```python
from build123d import *

# Parameters (mm, degrees)
F0_R     = 1.9
F1_DEPTH = 8
F2_R     = 2.9
F3_DEPTH = 10
F5_W     = 18.789151
F5_H     = 32.01971
F6_DEPTH = 25


with BuildPart() as f1:
    # F0 (on Top) → F1 (new body)
    with BuildSketch(Plane.XY):
        Circle(F0_R)
    extrude(amount=F1_DEPTH)

    # F2 (on face) → F3 (join)
    with BuildSketch(Plane(origin=(0, 0, 0), x_dir=(1, 0, 0), z_dir=(0, 0, -1))):
        Circle(F2_R)
    extrude(amount=F3_DEPTH)

    # F5 (on offset) → F6 (cut)
    with BuildSketch(Plane.XZ.offset(1.9)):
        with Locations((0.467039, -0.190436)):
            Rectangle(F5_W, F5_H)
    extrude(amount=F6_DEPTH, mode=Mode.SUBTRACT)


solid = f1.part
```
Design review of the part built by this model. Coordinates are the model's own, in mm. A direction names the side the tool comes from. Give positions to 0.01 mm unless a question says otherwise; leave off trailing zeros. Write each loop counter-clockwise with the first axis right and the second up, starting at its lowest first coordinate (ties: lowest second). Pieces come first, ordered by that corner, then holes.
(1) Add section B-B (x = 1.6). Give the boundary of the cut face in (y, z), and give its area (3 significant figures).
Checked values:
outline: (-1.9, -10) - (2.42, -10) - (2.42, 0) - (1.02, 0) - (1.02, 8) - (-1.02, 8) - (-1.02, 0) - (-1.9, 0) - close
area: 59.6 mm2
(2) Clearance check with flat-ended pins moving along their axes: pin 1 Ø2 at (y, z) = (0.5, -2.5) entering from -X; pin 2 Ø1.5 at (x, y) = (-2, 2.5) entering from +Z; pin 3 Ø1 at (x, z) = (2, 4) entering from +Y. State where each tip first meets the part, or that it passes through.
Checked values:
pin 1: stops at x = -2.9
pin 2: stops at z = 0
pin 3: stops at y = 1.17
(3) Tool access review of faces 1 (the face through (-1.9, 0.08, 3.94)), 2 (the face through (0, 0, 8)): name each direction out of +Z, -Z, +X, -X, +Y, -Y from which nothing blocks a thin tool from reaching the whole face with its end or side.
Checked values:
face 1: +Z
face 2: +Z, +X, -X, +Y, -Y
(4) Wall thickness on line 1 along Z through (x, y) = (2.3, 0.7); line 2 along Y through (x, z) = (-1.65, -5.5); line 3 along X through (y, z) = (1.35, 3.25): over which ranges is each line inside the solid? List them lowest first.
Checked values:
line 1: z = -10 to 0
line 2: y = -1.9 to 2.38
line 3: x = -1.34 to 1.34
(5) Add section D-D (z = 2.75). Give the boundary of the cut face in (x, y), and give its area (3 significant figures).
Checked values:
outline: circle Ø3.8 at (0, 0)
area: 11.3 mm2
(6) Add section A-A (y = 0). Give the boundary of the cut face in (x, z), and give its area (3 significant figures).
Checked values:
outline: (-2.9, -10) - (2.9, -10) - (2.9, 0) - (1.9, 0) - (1.9, 8) - (-1.9, 8) - (-1.9, 0) - (-2.9, 0) - close
area: 88.4 mm2
(7) Add section C-C (z = -2.75). Give the boundary of the cut face in (x, y), and give its area (3 significant figures).
Checked values:
outline: (-2.19, -1.9) - (2.19, -1.9) arc R2.9 ccw (long way) to start
area: 23.4 mm2
